```python
from build123d import *

# Parameters (mm, degrees)
SZKIC1_R                    = 47.5
DODANIE_WYCI_GNI_CIE1_DEPTH = 30
WYTNIJ_WYCI_GNI_CIE1_REACH  = 75.57
SZKIC2_R                    = 5
SZYK_KO_OWY1_COUNT          = 6
SZKIC3_R                    = 21
DODANIE_WYCI_GNI_CIE2_DEPTH = 0.001
SZKIC5_R                    = 22
DODANIE_WYCI_GNI_CIE4_DEPTH = 3
SZKIC7_R                    = 21
DODANIE_WYCI_GNI_CIE5_DEPTH = 15
DODANIE_WYCI_GNI_CIE6_DEPTH = 6.5
SZKIC14_W                   = 36.932370626
SZKIC14_H                   = 10
DODANIE_WYCI_GNI_CIE7_DEPTH = 10
ZAOKR_GLENIE1_R             = 7
ZAOKR_GLENIE2_R             = 7
ZAOKR_GLENIE3_R             = 5
WYTNIJ_WYCI_GNI_CIE2_REACH  = 130.377
SZKIC16_R                   = 11


# Read off the part's stored shape, not the designer's step: Lustro1
with BuildPart() as part:
    # Szkic1 → Dodanie-wyciągnięcie1 (new body)
    with BuildSketch(Plane.XY):
        Circle(SZKIC1_R)
    extrude(amount=DODANIE_WYCI_GNI_CIE1_DEPTH)

    # Szkic2 → Wytnij-wyciągnięcie1 (cut, up to next)
    with BuildSketch(Plane.XY.offset(30), mode=Mode.PRIVATE) as wytnij_wyci_gni_cie1_sk1:
        with Locations((0, 41.25)):
            Circle(SZKIC2_R)
    wytnij_wyci_gni_cie1_tool1 = extrude(wytnij_wyci_gni_cie1_sk1.sketch, amount=-WYTNIJ_WYCI_GNI_CIE1_REACH, mode=Mode.PRIVATE) & part.part
    wytnij_wyci_gni_cie1 = wytnij_wyci_gni_cie1_tool1.solids().sort_by_distance((0, 41.25, 30))[0]
    add(wytnij_wyci_gni_cie1, mode=Mode.SUBTRACT)

    # Szyk kołowy1: Wytnij-wyciągnięcie1 ×6 about axis
    szyk_ko_owy1_axis = Axis((0, 0, 0), (0, 0, 1))
    for i in range(1, SZYK_KO_OWY1_COUNT):
        add(wytnij_wyci_gni_cie1.rotate(szyk_ko_owy1_axis, i * 360 / SZYK_KO_OWY1_COUNT), mode=Mode.SUBTRACT)

    # Szkic3 → Dodanie-wyciągnięcie2 (add)
    with BuildSketch(Plane.XY.offset(30)):
        Circle(SZKIC3_R)
    extrude(amount=DODANIE_WYCI_GNI_CIE2_DEPTH)

    # Szkic5 → Dodanie-wyciągnięcie4 (add)
    with BuildSketch(Plane.XY.offset(30.001)):
        Circle(SZKIC5_R)
    extrude(amount=DODANIE_WYCI_GNI_CIE4_DEPTH)

    # Szkic7 → Dodanie-wyciągnięcie5 (add)
    with BuildSketch(Plane.XY.offset(33.001)):
        Circle(SZKIC7_R)
    extrude(amount=DODANIE_WYCI_GNI_CIE5_DEPTH)

    # Szkic9 → Dodanie-wyciągnięcie6 (add, symmetric)
    with BuildSketch(Plane(origin=(0, 26.5, 0), x_dir=(1, 0, 0), z_dir=(0, 1, 0))):
        Polygon((-20.374433176, -38.001), (-16, -88.001), (16, -88.001), (20.374433176, -38.001), align=None)
    extrude(amount=DODANIE_WYCI_GNI_CIE6_DEPTH, both=True)

    # Szkic14 → Dodanie-wyciągnięcie7 (add)
    with BuildSketch(Plane(origin=(0, 10, 0), x_dir=(1, 0, 0), z_dir=(0, 1, 0))):
        with Locations((0, -43.001)):
            Rectangle(SZKIC14_W, SZKIC14_H)
    extrude(amount=DODANIE_WYCI_GNI_CIE7_DEPTH)

    # Zaokrąglenie1
    # the kernel refuses this fillet: 7 mm, written as the material it adds along each edge
    with BuildSketch(Plane(origin=(0, 0, 38.001), x_dir=(-0.9435381877974668, -0.33126377430662785, 0), z_dir=(0.33126377430662785, -0.9435381877974668, 0))) as zaokr_glenie1_piece_1_section:
        with BuildLine():
            CenterArc((21 + ZAOKR_GLENIE1_R, ZAOKR_GLENIE1_R), ZAOKR_GLENIE1_R, 180, 90)
            Line((21 + ZAOKR_GLENIE1_R, 0), (21, 0))
            Line((21, 0), (21, ZAOKR_GLENIE1_R))
        make_face()
    zaokr_glenie1_piece_1 = revolve(axis=Axis((0, 0, 38.001), (0, 0, -1)), revolution_arc=218.690998802, mode=Mode.PRIVATE)
    zaokr_glenie1_piece_1 = split(zaokr_glenie1_piece_1, bisect_by=Plane(origin=(-18.694483681, 20, 37.992305912), z_dir=(0, 1, 0)), keep=Keep.TOP, mode=Mode.PRIVATE)
    add(zaokr_glenie1_piece_1)
    with BuildSketch(Plane(origin=(0, 0, 38.001), x_dir=(-0.9435381877974668, -0.33126377430662785, 0), z_dir=(0.33126377430662785, -0.9435381877974668, 0))) as zaokr_glenie1_piece_2_section:
        with BuildLine():
            CenterArc((21 + ZAOKR_GLENIE1_R, ZAOKR_GLENIE1_R), ZAOKR_GLENIE1_R, 180, 90)
            Line((21 + ZAOKR_GLENIE1_R, 0), (21, 0))
            Line((21, 0), (21, ZAOKR_GLENIE1_R))
        make_face()
    zaokr_glenie1_piece_2 = revolve(axis=Axis((0, 0, 38.001), (0, 0, -1)), revolution_arc=218.690998802, mode=Mode.PRIVATE)
    zaokr_glenie1_piece_2 = split(zaokr_glenie1_piece_2, bisect_by=Plane(origin=(-18.466185313, 16.543060956, 36.276393693), z_dir=(1, 0, 0)), keep=Keep.TOP, mode=Mode.PRIVATE)
    zaokr_glenie1_piece_2 = split(zaokr_glenie1_piece_2, bisect_by=Plane(origin=(18.466185313, 16.543060956, 36.276393693), z_dir=(-1, 0, 0)), keep=Keep.TOP, mode=Mode.PRIVATE)
    add(zaokr_glenie1_piece_2)
    with BuildSketch(Plane(origin=(18.466185313, 20, 48.001), x_dir=(0, 0, 1), z_dir=(-1, 0, 0))) as zaokr_glenie1_piece_3:
        with BuildLine():
            CenterArc((ZAOKR_GLENIE1_R, -ZAOKR_GLENIE1_R), ZAOKR_GLENIE1_R, 90, 90)
            Line((0, -ZAOKR_GLENIE1_R), (0, 0))
            Line((0, 0), (ZAOKR_GLENIE1_R, 0))
        make_face()
    extrude(amount=36.932370625)

    # Zaokrąglenie2
    zaokr_glenie2_edges = [part.edges().sort_by_distance(p)[0] for p in [
        (0, 33, 38.001),
    ]]
    fillet(zaokr_glenie2_edges, radius=ZAOKR_GLENIE2_R)

    # Zaokrąglenie3
    zaokr_glenie3_edges = [part.edges().sort_by_distance(p)[0] for p in [
        (0, 20, 88.001),
        (-16, 26.5, 88.001),
        (16, 26.5, 88.001),
        (0, 33, 88.001),
    ]]
    fillet(zaokr_glenie3_edges, radius=ZAOKR_GLENIE3_R)

    # Szkic16 → Wytnij-wyciągnięcie2 (cut, up to next)
    with BuildSketch(Plane(origin=(0, 33, 0), x_dir=(1, 0, 0), z_dir=(0, 1, 0)), mode=Mode.PRIVATE) as wytnij_wyci_gni_cie2_sk1:
        with Locations(Location((0, -68.001, 0), (0, 0, 270))):
            Circle(SZKIC16_R)
    wytnij_wyci_gni_cie2_tool1 = extrude(wytnij_wyci_gni_cie2_sk1.sketch, amount=-WYTNIJ_WYCI_GNI_CIE2_REACH, mode=Mode.PRIVATE) & part.part
    add(wytnij_wyci_gni_cie2_tool1.solids().sort_by_distance((0, 33, 68.001))[0], mode=Mode.SUBTRACT)

    # Lustro1: part across plane


with BuildPart() as part_1:
    add(part.part)
    add(part.part.mirror(Plane.ZX))


solid = part_1.part
```
The model under review builds one solid part; all positions refer to its coordinate system, in mm. A direction names the side the tool comes from. Coordinates: 2 decimals unless noted, no trailing zeros. Loops run counter-clockwise (first coordinate to the right, second up) from the corner with the lowest first, then second, coordinate; pieces in that order, holes last. Notation, with made-up numbers: (59, 36.5) -> (81, 36.5) arc R15 cw to (81, 65.5) -> close; hole circle Ø4 at (33.25, -35). An arc over 180 degrees is marked (long way). Answer as CSV lines item,"result".
Item 1: Insertion check: pin 1 (10 mm diameter, centred on y = 2, z = 20, fed in from +X); pin 2 (12 mm diameter, centred on x = -6, y = -37.5, fed in from +Z); pin 3 (19 mm diameter, centred on x = -4.5, z = 64, fed in from +Y); pin 4 (10 mm diameter, centred on x = 7.5, z = 27, fed in from -Y). Each pin has a flat end and moves straight along its axis. Give the tip position at first contact, or say it passes through.
Results below:
pin 1,"stops at x = 47.5"
pin 2,"stops at z = 86.57"
pin 3,"stops at y = 33"
pin 4,"stops at y = -47.43"
Item 2: Take a section at B-B, the plane z = 67. State the section outline as (x, y) points, and give its area (3 significant figures).
Results below:
outline,"(-17.84, -33) -> (-10.95, -33) -> (-10.95, -20) -> (-17.84, -20) -> close; (-17.84, 20) -> (-10.95, 20) -> (-10.95, 33) -> (-17.84, 33) -> close; (10.95, -33) -> (17.84, -33) -> (17.84, -20) -> (10.95, -20) -> close; (10.95, 20) -> (17.84, 20) -> (17.84, 33) -> (10.95, 33) -> close"
area,"358 mm2"
Item 3: Draft analysis for pull direction Y (two halves, no side actions). For faces 1 (the cylindrical face through (0, 27, 57)), 2 (the cylindrical face through (-15.5, 30.9, 40)), 3 (the flat face through (18.466, 15, 42)), 4 (the cylindrical face through (-10.3, -46.37, 14.79)), state which applies: +Y half, -Y half, draft (parallel to the pull), parting line (faces both ways), or undercut.
Results below:
face 1,"draft"
face 2,"+Y half"
face 3,"undercut"
face 4,"parting line"
Item 4: Take a section at D-D, the plane x = 35. State the section outline as (y, z) points, and give its area (3 significant figures).
Results below:
outline,"(-32.11, 0) -> (-25.57, 0) -> (-25.57, 30) -> (-32.11, 30) -> close; (-15.68, 0) -> (15.68, 0) -> (15.68, 30) -> (-15.68, 30) -> close; (25.57, 0) -> (32.11, 0) -> (32.11, 30) -> (25.57, 30) -> close"
area,"1,330 mm2"
Item 5: Machinability: for faces 5 (the flat face through (18.36, 26.59, 61.04)), 6 (the flat face through (-18, 24, 38.001)), 7 (the flat face through (-18, -24, 38.001)), 8 (the flat face through (0, 0, 48.001)), 9 (the flat face through (-18.466, 15, 42)), which of the approach directions +Z, -Z, +X, -X, +Y, -Y give a long, thin tool a straight path to every point of the face, cutting with its end or side? Answer none if there is none.
Results below:
face 5,"+Z, +X, +Y"
face 6,"-X, +Y"
face 7,"-X, -Y"
face 8,"+Z, +X, -X"
face 9,"+Z, -X"
Item 6: Take a section at C-C, the plane z = 7.5. State the section outline as (x, y) points (3 decimals).
Results below:
outline,"circle Ø95 at (0, 0); hole circle Ø10 at (-35.724, -20.625); hole circle Ø10 at (-35.724, 20.625); hole circle Ø10 at (0, -41.25); hole circle Ø10 at (0, 41.25); hole circle Ø10 at (35.724, -20.625); hole circle Ø10 at (35.724, 20.625)"
Item 7: For L1, parallel to Y at x = 4.5, z = 8; L2, parallel to X at y = 41, z = 11; L3, parallel to Z at x = 11, y = -11, list the stretches that pass through material, from the lowest coordinate up.
Results below:
L1,"y = -47.29 to -43.43, -39.07 to 39.07, 43.43 to 47.29"
L2,"x = -23.98 to -4.99, 4.99 to 23.98"
L3,"z = 0 to 48"
